from build123d import *

# Parameters (mm, degrees)
EXTRUDE_1_DEPTH     = 8
SKETCH_3_W          = 6
SKETCH_3_H          = 30
CUT_EXTRUDE_2_DEPTH = 2.1
CUT_EXTRUDE_3_DEPTH = 68.186308129
FILLET_1_R          = 2
FILLET_2_R          = 5


with BuildPart() as part:
    # 草图1 → 凸台-拉伸1 (new body)
    with BuildSketch(Plane.XY):
        with BuildLine():
            Line((-11.1, -4.1), (-11.1, -15))
            Line((-11.1, -15), (-32.5, -15))
            Line((-32.5, -15), (-32.5, 15))
            Line((-32.5, 15), (32.5, 15))
            Line((32.5, 15), (32.5, -15))
            Line((32.5, -15), (11.1, -15))
            Line((11.1, -15), (11.1, -4.1))
            ThreePointArc((11.1, -4.1), (0, 7), (-11.1, -4.1))
        make_face()
    extrude(amount=EXTRUDE_1_DEPTH)

    # 草图3 → 切除-拉伸2 (cut)
    with BuildSketch(Plane.XY.offset(8)):
        with Locations((-13.5, 0)):
            Rectangle(SKETCH_3_W, SKETCH_3_H)
        with Locations((13.5, 0)):
            Rectangle(SKETCH_3_W, SKETCH_3_H)
    extrude(amount=-CUT_EXTRUDE_2_DEPTH, mode=Mode.SUBTRACT)

    # 草图2 → 切除-拉伸3 (cut, through all)
    with BuildSketch(Plane(origin=(32.5, 0, 0), x_dir=(0, 0, -1), z_dir=(1, 0, 0))):
        Polygon((-4, -15), (-8, -4.1), (-8, -15), align=None)
    extrude(amount=-CUT_EXTRUDE_3_DEPTH, mode=Mode.SUBTRACT)

    # 圆角1
    fillet_1_edges = [part.edges().sort_by_distance(p)[0] for p in [
        (-32.5, 0, 0),
        (0, 15, 0),
        (32.5, 0, 0),
        (24.5, 15, 8),
        (-32.5, 15, 4),
        (32.5, 15, 4),
        (-32.5, 5.45, 8),
        (0, 15, 8),
        (-24.5, 15, 8),
        (-10.5, 7.25, 8),
        (-16.5, 5.45, 8),
        (10.5, 7.25, 8),
        (16.5, 5.45, 8),
        (11.1, -15, 2),
        (-32.5, -15, 2),
        (-11.1, -15, 2),
        (32.5, 5.45, 8),
        (32.5, -15, 2),
        (21.8, -15, 4),
        (-21.8, -15, 4),
    ]]
    fillet(fillet_1_edges, radius=FILLET_1_R)

    # 圆角2
    # the kernel refuses this fillet: 5 mm, written as the material it takes off along each edge
    with BuildSketch(Plane(origin=(32.721158942, -4.1, 8), x_dir=(0, -0.9387834907734438, -0.34450770303612566), z_dir=(-1, 0, 0)), Plane(origin=(-16.278841058, -4.1, 8), x_dir=(0, -0.9387834907734438, -0.34450770303612566), z_dir=(-1, 0, 0))) as fillet_2_piece_1:
        with BuildLine():
            CenterArc((FILLET_2_R * 0.177692715394, -FILLET_2_R), FILLET_2_R, 90, 20.151747034)
            Line((-FILLET_2_R * 0.166814987642, -FILLET_2_R * 0.0612165092266), (0, 0))
            Line((0, 0), (FILLET_2_R * 0.177692715394, 0))
        make_face()
    extrude(amount=16.442317885, mode=Mode.SUBTRACT)


solid = part.part
For this review, take the finished solid that the model builds, in its own axes (mm). A direction names the side the tool comes from. Coordinates: 2 decimals unless noted, no trailing zeros. Loops run counter-clockwise (first coordinate to the right, second up) from the corner with the lowest first, then second, coordinate; pieces in that order, holes last. Notation, with made-up numbers: (-19.75, 13) -> (36.25, 13) arc R10 ccw to (36.25, 31) -> close; hole circle Ø2 at (-1.75, -15). An arc over 180 degrees is marked (long way). Write each question's results on one line, items separated by ' | '.
Q1. Add section D-D, the plane x = 12. State the section outline as (y, z) points, then the cut area to 3 significant figures.
Taken from the geometry:
outline: (-14.67, 0) -> (13, 0) arc R2 ccw to (15, 2) -> (15, 5.9) -> (-9.82, 5.9) -> (-13.69, 4.48) arc R2 ccw to (-14.67, 3.7) -> close | area: 170 mm²
Q2. Mouldability with a two-part tool opening along X and no side actions: class faces 4 (the cylindrical face through (-31.93, 14.4, 4.03)), 5 (the flat face through (0, 9, 8)), 6 (the flat face through (11.1, -9, 3)) as +X half, -X half, draft (parallel to the pull), parting line (faces both ways), or undercut.
Taken from the geometry:
face 4: -X half | face 5: draft | face 6: undercut
Q3. Add section C-C, the plane y = 5.5. State the section outline as (x, z) points, then the cut area to 3 significant figures.
Taken from the geometry:
outline: (-32.5, 2) arc R2 ccw to (-30.5, 0) -> (-5.57, 0) -> (-5.57, 8) -> (-8.5, 8) arc R2 ccw to (-10.5, 6) -> (-10.5, 5.9) -> (-16.5, 5.9) -> (-16.5, 6) arc R2 ccw to (-18.5, 8) -> (-30.5, 8) arc R2 ccw to (-32.5, 6) -> close; (5.57, 0) -> (30.5, 0) arc R2 ccw to (32.5, 2) -> (32.5, 6) arc R2 ccw to (30.5, 8) -> (18.5, 8) arc R2 ccw to (16.5, 6) -> (16.5, 5.9) -> (10.5, 5.9) -> (10.5, 6) arc R2 ccw to (8.5, 8) -> (5.57, 8) -> close | area: 399 mm²
Q4. Add section A-A, the plane y = 11. State the section outline as (x, z) points.
Taken from the geometry:
outline: (-32.5, 2) arc R2 ccw to (-30.5, 0) -> (30.5, 0) arc R2 ccw to (32.5, 2) -> (32.5, 6) arc R2 ccw to (30.5, 8) -> (18.5, 8) arc R2 ccw to (16.5, 6) -> (16.5, 5.9) -> (10.5, 5.9) -> (10.5, 6) arc R2 ccw to (8.5, 8) -> (-8.5, 8) arc R2 ccw to (-10.5, 6) -> (-10.5, 5.9) -> (-16.5, 5.9) -> (-16.5, 6) arc R2 ccw to (-18.5, 8) -> (-30.5, 8) arc R2 ccw to (-32.5, 6) -> close
Q5. Machinability: for faces 1 (the cylindrical face through (9.9, 7.36, 7.43)), 2 (the flat face through (-24.028, -9.373, 6.065)), 3 (the cylindrical face through (11.7, -14.43, 1.87)), which of the approach directions +Z, -Z, +X, -X, +Y, -Y give a long, thin tool a straight path to every point of the face, cutting with its end or side? Answer none if there is none.
Taken from the geometry:
face 1: +Z, +Y, -Y | face 2: +Z, +X, -X, -Y | face 3: +Z, -Z, -Y
Q6. For pin 1 Ø6.5 at (x, y) = (15, 2) entering from +Z; pin 2 Ø3 at (y, z) = (-10, 1.5) entering from -X; pin 3 Ø8 at (x, y) = (10, -3) entering from +Z, all flat-tipped, find the tip position at first contact; note any pin that passes through.
Taken from the geometry:
pin 1: z = 7.98 | pin 2: x = -32.5 | pin 3: z = 7.47
Q7. To check wall thickness, follow line 1 along X through (y, z) = (-6, 3.5); line 2 along Y through (x, z) = (-8.5, 2.5); line 3 along X through (y, z) = (8, 7.75). State the ranges of each line that lie inside material, in increasing order. Write a range as [from, to].
Taken from the geometry:
line 1: [-32.5, -11.1], [11.1, 32.5] | line 2: [3.04, 15] | line 3: [-31.47, -17.53], [-9.47, 9.47], [17.53, 31.47]
Q8. Add section B-B, the plane x = 0. State the section outline as (y, z) points.
Taken from the geometry:
outline: (7, 0) -> (13, 0) arc R2 ccw to (15, 2) -> (15, 6) arc R2 ccw to (13, 8) -> (7, 8) -> close
